```python
from build123d import *

# Parameters (mm, degrees)
SKETCH1_W             = 150
SKETCH1_H             = 50
BOSS_EXTRUDE2_DEPTH   = 150
BOSS_EXTRUDE2_2_DEPTH = 150
SKETCH1_4_R           = 37.5
SKETCH1_4_W           = 150
SKETCH1_4_H           = 50
BOSS_EXTRUDE3_DEPTH   = 50
FILLET2_RADIUS        = 75
FILLET2_LENGTH        = 50
FILLET3_RADIUS        = 75
FILLET3_LENGTH        = 50
SKETCH2_R             = 37.5
CUT_EXTRUDE1_DEPTH    = 576.129630886
SKETCH3_R             = 37.5
CUT_EXTRUDE2_DEPTH    = 598.441520826


with BuildPart() as part:
    # Sketch1 → Boss-Extrude2 (new body)
    with BuildSketch(Plane.XY):
        with Locations((75, 25)):
            Rectangle(SKETCH1_W, SKETCH1_H)
    extrude(amount=BOSS_EXTRUDE2_DEPTH)



with BuildPart() as body_2:
    # Sketch1 → Boss-Extrude2 2 (new body)
    with BuildSketch(Plane.XY):
        Polygon((358.253175473, 105.801270189), (383.253175473, 62.5), (513.156986041, 137.5), (488.156986041, 180.801270189), align=None)
    extrude(amount=BOSS_EXTRUDE2_2_DEPTH)


with BuildPart() as part_1:
    add(part.part)

    add(body_2.part)  # Boss-Extrude3 merges body 2
    # Sketch1<4> → Boss-Extrude3 (add)
    # profile 1 of 3: a face of its own
    with BuildSketch(Plane.XY):
        with BuildLine():
            Line((150, 50), (150, 0))
            Line((150, 0), (275, 0))
            Line((275, 0), (383.253175473, 62.5))
            Line((383.253175473, 62.5), (358.253175473, 105.801270189))
            Line((358.253175473, 105.801270189), (291.750893275, 220.986601776))
            ThreePointArc((291.750893275, 220.986601776), (207.419297449, 259.935945937), (149.893501015, 187))
            Line((149.893501015, 187), (149.89359166, 186.883395343))
            Line((149.89359166, 186.883395343), (150, 50))
        make_face()
        with Locations((224.893501015, 187)):
            Circle(SKETCH1_4_R, mode=Mode.SUBTRACT)
    # profile 2 of 3: a face of its own
    with BuildSketch(Plane.XY):
        with Locations((75, 25)):
            Rectangle(SKETCH1_4_W, SKETCH1_4_H)
    # profile 3 of 3: a face of its own
    with BuildSketch(Plane.XY):
        Polygon((358.253175473, 105.801270189), (383.253175473, 62.5), (513.156986041, 137.5), (488.156986041, 180.801270189), align=None)
    extrude(amount=BOSS_EXTRUDE3_DEPTH)

    # Fillet2: full round fillet: the end face becomes a half cylinder, R = half its width
    fillet2_face = Plane((435.705080757, 121.650635095, 150), x_dir=(0.5, -0.866025403784, 0), z_dir=(0, 0, 1))  # on the end face: x along it, z out of the body
    fillet2_slab = fillet2_face.offset(-FILLET2_RADIUS / 2) * Box(FILLET2_LENGTH, 2 * FILLET2_RADIUS, FILLET2_RADIUS, mode=Mode.PRIVATE)  # the body's end, R deep
    fillet2_round = Plane((435.705080757, 121.650635095, 75), x_dir=(0, 0, 1), z_dir=(0.5, -0.866025403784, 0)) * Cylinder(FILLET2_RADIUS, FILLET2_LENGTH, mode=Mode.PRIVATE)  # its axis R under the face
    add(fillet2_slab - fillet2_round, mode=Mode.SUBTRACT)

    # Fillet3: full round fillet: the end face becomes a half cylinder, R = half its width
    fillet3_face = Plane((75, 25, 150), x_dir=(0, -1, 0), z_dir=(0, 0, 1))  # on the end face: x along it, z out of the body
    fillet3_slab = fillet3_face.offset(-FILLET3_RADIUS / 2) * Box(FILLET3_LENGTH, 2 * FILLET3_RADIUS, FILLET3_RADIUS, mode=Mode.PRIVATE)  # the body's end, R deep
    fillet3_round = Plane((75, 25, 75), x_dir=(0, 0, 1), z_dir=(0, -1, 0)) * Cylinder(FILLET3_RADIUS, FILLET3_LENGTH, mode=Mode.PRIVATE)  # its axis R under the face
    add(fillet3_slab - fillet3_round, mode=Mode.SUBTRACT)

    # Sketch2 → Cut-Extrude1 (cut, through all)
    with BuildSketch(Plane(origin=(0, 50, 0), x_dir=(1, 0, 0), z_dir=(0, 1, 0))):
        with Locations(Location((75, -75, 0), (0, 0, 270))):
            Circle(SKETCH2_R)
    extrude(amount=-CUT_EXTRUDE1_DEPTH, mode=Mode.SUBTRACT)

    # Sketch3 → Cut-Extrude2 (cut, through all)
    with BuildSketch(Plane(origin=(43.75, -75.777222831, 0), x_dir=(0.8660254037844382, 0.500000000000001, 0), z_dir=(-0.500000000000001, 0.8660254037844382, 0))):
        with Locations(Location((438.156986041, -75, 0), (0, 0, 180))):
            Circle(SKETCH3_R)
    extrude(amount=-CUT_EXTRUDE2_DEPTH, mode=Mode.SUBTRACT)


solid = part_1.part
```
Source: CAD feature listing. Evaluate the final solid. Frame: model axes, mm. A direction names the side the tool comes from. Give positions to 0.01 mm unless a question says otherwise; leave off trailing zeros. Loops run counter-clockwise (first coordinate to the right, second up) from the corner with the lowest first, then second, coordinate; pieces in that order, holes last. Notation, with made-up numbers: (6.25, 82) -> (12.25, 82) arc R33 ccw to (12.25, 112) -> close; hole circle Ø1 at (75, -29). An arc over 180 degrees is marked (long way). Put each result on its own line as item: value. Start each with the question number.
1) Cut plane A-A (x = 75). Return loops of the section in (y, z).
2) Cut plane D-D (y = 31). Return loops of the section in (x, z).
3) Cut plane C-C (y = 214). Return loops of the section in (x, z), then the cut area to 3 significant figures.
4) Material intervals for probe 1 along X at (y, z) = (23, 75); probe 2 along Z at (x, y) = (218, 23); probe 3 along Y at (x, z) = (226.5, 12), sorted ascending.
5) Reachability of faces 4 (the face through (150, 25, 62)), 5 (the face through (325.468, 162.588, 24.65)), 6 (the face through (57, 50, 41)), 7 (the face through (370.58, 84.45, 62.32)) from +Z, -Z, +X, -X, +Y, -Y: full face, straight path, thin tool, end or side. Return the list, or none.
6) Cut plane B-B (z = 107). Return loops of the section in (x, y), then the cut area to 3 significant figures.
7) Contact query for flat-ended pins moving along their axis: P1, Ø10, axis at y = 83, z = 105.5, coming from the -X side; P2, Ø2, axis at x = 243, z = 37, coming from the +Y side; P3, Ø1.5, axis at x = 245, z = 49, coming from the +Y side. Output: stop coordinate, or through.
8) Draft query along Y for faces 1 (the face through (86.26, 25.35, 110.77)), 2 (the face through (260.662, 198.264, 24.65)), 3 (the face through (409.681, 135.493, 40.617)). Return one class per face: released by +Y, released by -Y, zero draft, split by the parting line, or undercut.
Results are:
1. outline: (0, 0) -> (50, 0) -> (50, 37.5) -> (0, 37.5) -> close; (0, 112.5) -> (50, 112.5) -> (50, 150) -> (0, 150) -> close
2. outline: (0, 0) -> (328.69, 0) -> (328.69, 50) -> (150, 50) -> (150, 75) arc R75 ccw to (0, 75) -> close; hole circle Ø75 at (75, 75)
3. outline: (154.92, 0) -> (198.87, 0) -> (198.87, 50) -> (154.92, 50) -> close; (250.92, 0) -> (295.78, 0) -> (295.78, 50) -> (250.92, 50) -> close
3. area: 4,440 mm2
4. probe 1: x = 0 to 37.5, 112.5 to 150
4. probe 2: z = 0 to 50
4. probe 3: y = 0 to 149.53, 224.47 to 261.98
5. face 4: +Z, +X, +Y, -Y
5. face 5: +Z, -Z, +Y
5. face 6: +Z, -Z, -X, +Y
5. face 7: +Z, -X, -Y
6. outline: (7.17, 0) -> (55.45, 0) -> (55.45, 50) -> (7.17, 50) -> close; (94.55, 0) -> (142.83, 0) -> (142.83, 50) -> (94.55, 50) -> close; (364.46, 109.39) -> (389.46, 66.08) -> (431.27, 90.22) -> (406.27, 133.53) -> close; (440.14, 153.08) -> (465.14, 109.78) -> (506.95, 133.92) -> (481.95, 177.22) -> close
6. area: 9,660 mm2
7. P1: stops at x = 375.14
7. P2: stops at y = 260.02
7. P3: stops at y = 259.46
8. face 1: zero draft
8. face 2: undercut
8. face 3: released by +Y
